Autodesk Fusion 360 part; units mm, degrees
sketch "Sketch1" plane through (0, 0, 0) normal (0, 0, 1) x (1, 0, 0)
  circle A0 centre (0, 0) radius 6.5
  circle A1 centre (0, 0) radius 11
  line L0 (0, 0) -> (9, 0) construction
  line L1 (0, 0) -> (6.5, 0)
  line L2 (6.5, 0) -> (6.5, 3)
  line L3 (6.5, 3) -> (26.5, 3)
  line L4 (26.5, 3) -> (26.5, -3)
  line L5 (26.5, -3) -> (6.5, -3)
  line L6 (6.5, -3) -> (6.5, 3)
  dimension "d1" = 13
  dimension "d2" = 22
  dimension "d21" = 3
  dimension "d22" = 20
  dimension "d23" = 6
extrude "Extrude1" add sketch "Sketch1" along normal blind 10
hole "Hole1" at (26.5, 0, 2.5) direction (-1, 0, 0) diameter 1.623 depth 10 tip angle 118
hole "Hole3" at (-11, 0, 6.1111) direction (1, 0, 0) diameter 3.416 depth 10 tip angle 118
chamfer "Chamfer1" distance 0.25 angle 45 4 edges at (10.583, -3, 5) (10.583, 3, 5) (26.5, -3, 5) (26.5, 3, 5) 2 faces at (15.8887, -1, 10) (15.8887, -1, 0)
equation "d16 = ( 6 / 2 ) * 1 mm"
equation "d21 = d23 / 2"
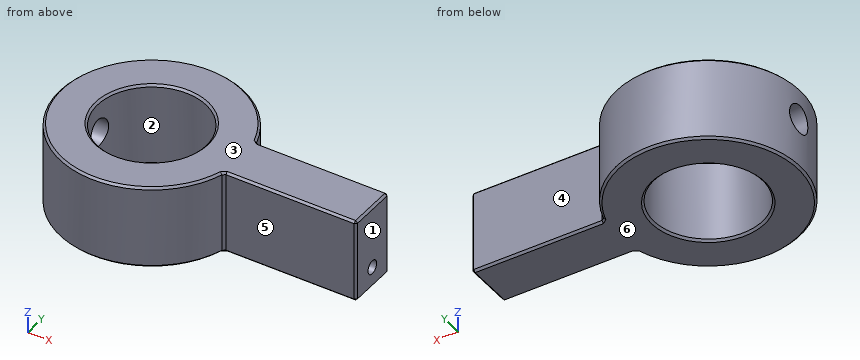
Verification items for the finished model (mm, model axes). Face numbers are marked on the shaded views. A direction names the side the tool comes from. Coordinates: 2 decimals unless noted, no trailing zeros. Order: outer loops, then holes, each group sorted by start corner. A loop starts at its lowest first (then second) coordinate and runs counter-clockwise, first axis right, second up.
Item 1: Section check C-C, the plane x = 14.5. Enter the section's corners in (y, z).
Filled in:
outline: (-3, 0.25) - (-2.75, 0) - (2.75, 0) - (3, 0.25) - (3, 9.75) - (2.75, 10) - (-2.75, 10) - (-3, 9.75) - close
Item 2: Depth check by flat-ended pin: pin 1 (3 mm diameter, centred on x = 14, z = 5.5, fed in from +Y); pin 2 (2 mm diameter, centred on x = -1.5, z = 4.5, fed in from -Y); pin 3 (2 mm diameter, centred on y = 8, z = 4.5, fed in from +X); pin 4 (4 mm diameter, centred on x = 18.5, y = 5.5, fed in from -Z). Enter the tip coordinate at first touch or a pass-through.
Filled in:
pin 1: stops at y = 3
pin 2: stops at y = -10.99
pin 3: stops at x = 8.49
pin 4: passes through
Item 3: Section check D-D, the plane x = 0. Enter the section's corners in (y, z), then the cut area to 4 significant figures.
Filled in:
outline: (-11, 0.25) - (-10.75, 0) - (-6.75, 0) - (-6.5, 0.25) - (-6.5, 9.75) - (-6.75, 10) - (-10.75, 10) - (-11, 9.75) - close; (6.5, 0.25) - (6.75, 0) - (10.75, 0) - (11, 0.25) - (11, 9.75) - (10.75, 10) - (6.75, 10) - (6.5, 9.75) - close
area: 89.75 mm2
Item 4: Section check B-B, the plane x = 24. Enter the section's corners in (y, z).
Filled in:
outline: (-3, 0.25) - (-2.75, 0) - (2.75, 0) - (3, 0.25) - (3, 9.75) - (2.75, 10) - (-2.75, 10) - (-3, 9.75) - close; hole circle Ø1.62 at (0, 2.5)
Item 5: Section check A-A, the plane z = 4. Enter the section's corners in (x, y), then the cut area to 3 significant figures.
Filled in:
outline: (10.51, -3.24) - (10.83, -3) - (26.25, -3) - (26.5, -2.75) - (26.5, 2.75) - (26.25, 3) - (10.83, 3) - (10.51, 3.24) arc R11 ccw (long way) to start; hole circle Ø13 at (0, 0)
area: 341 mm2
Item 6: Access from +Z, -Z, +X, -X, +Y, -Y to the whole of each face (thin tool, end or side, straight path). Record for the marked faces 4, 5 and 6.
Filled in:
face 4: +Z, -Z, +X, +Y
face 5: +Z, -Z, +X, -Y
face 6: -Z, +X, -X, +Y, -Y
Item 7: Release check for a two-part mould opening along X. For the marked faces 1, 2 and 3 record: +X half, -X half, draft (parallel to the pull), parting line (faces both ways), or undercut.
Filled in:
face 1: +X half
face 2: undercut
face 3: draft
Item 8: Material ranges on L1, parallel to Z at x = 22.5, y = 0; L2, parallel to Y at x = 21.25, z = 2.5; L3, parallel to Y at x = 17, z = 4.5, recorded low to high.
Filled in:
L1: z = 0 to 1.69, 3.31 to 10
L2: y = -3 to -0.81, 0.81 to 3
L3: y = -3 to 3
